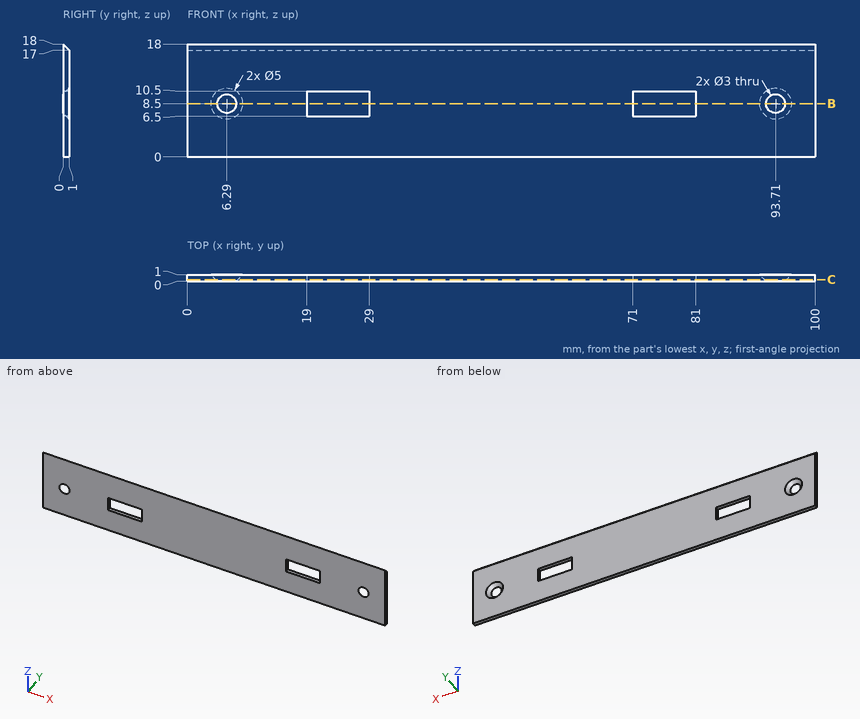
Geometry check sheet. Reference: drawing and pictorial views, mm from the part's lowest x, y, z. Coordinates: 2 decimals unless noted, no trailing zeros. Loops run counter-clockwise (first coordinate to the right, second up) from the corner with the lowest first, then second, coordinate; pieces in that order, holes last.
1) Sectioned sample at C-C (y = 0.25). Record the boundary of the cut face in (x, z).
2) Material ranges on probe 1 along Z at (x, y) = (78, 0.1); probe 2 along Z at (x, y) = (31, 0.9); probe 3 along Z at (x, y) = (70.5, 0.25), recorded low to high.
3) Gauge pin test, flat ends, axial feed: pin 1 (0.5 mm diameter, centred on x = 77.5, y = 0.5, fed in from -Z); pin 2 (0.5 mm diameter, centred on x = 22.5, y = 0.5, fed in from +Z). Record the tip position at first contact, or that the pin passes through.
4) Sectioned sample at B-B (z = 8.5). Count the separate pieces of the cut face and the enclosed holes in it.
Check sheet entries:
1. outline: (0, 0) - (100, 0) - (100, 17.75) - (0, 17.75) - close; hole circle Ø3.5 at (6.29, 8.5); hole (19, 6.5) - (29, 6.5) - (29, 10.5) - (19, 10.5) - close; hole (71, 6.5) - (81, 6.5) - (81, 10.5) - (71, 10.5) - close; hole circle Ø3.5 at (93.71, 8.5)
2. probe 1: z = 0 to 6.5, 10.5 to 17.9
2. probe 2: z = 0 to 17.1
2. probe 3: z = 0 to 17.75
3. pin 1: stops at z = 0
3. pin 2: stops at z = 17.75
4. separate pieces: 5
4. enclosed holes: 0
